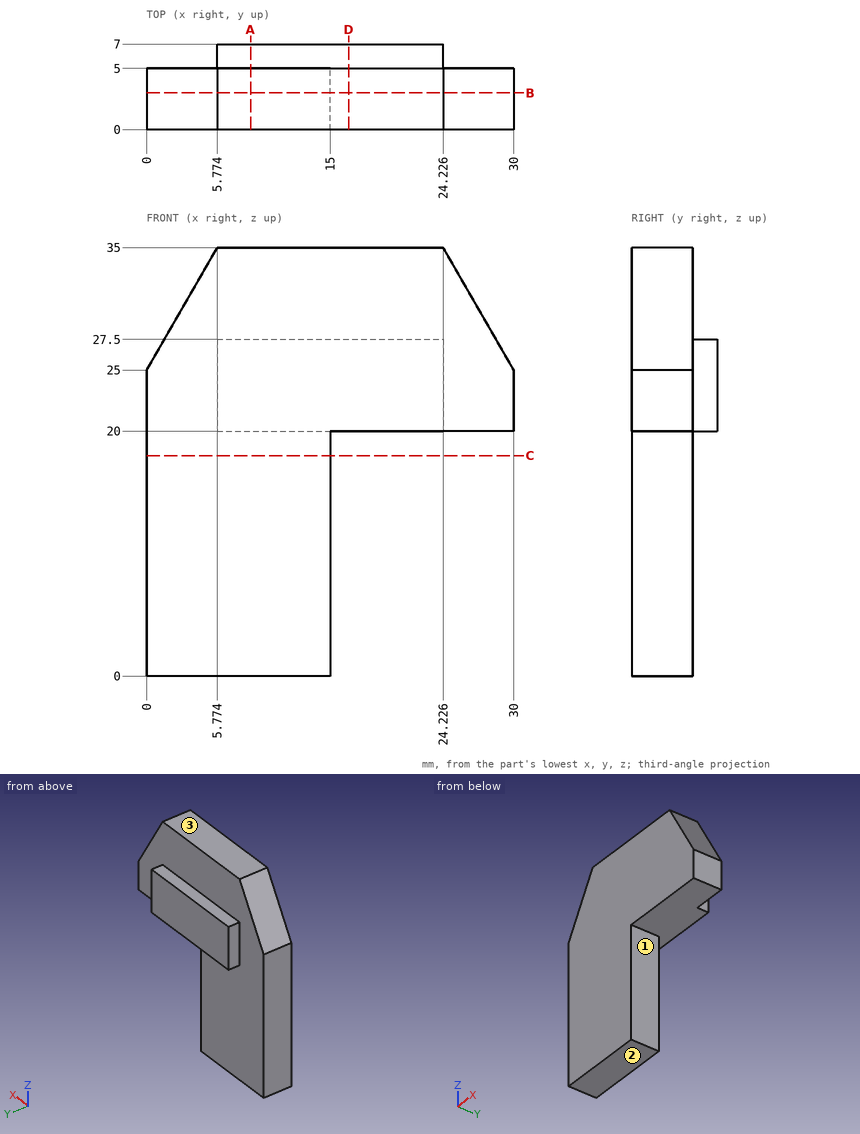
Verification items for this drawing (mm, ordinates from the low corner). Coordinates: 2 decimals unless noted, no trailing zeros. Order: outer loops, then holes, each group sorted by start corner. A loop starts at its lowest first (then second) coordinate and runs counter-clockwise, first axis right, second up. Notation, with made-up numbers: M 81,22 L 91,22 A18 ccw 91,57 Z; hole C 87.25,39.5 d7. An arc over 180 degrees is marked long. One line per item, written item: value. Start each with the question number.
Item 1: Thickness scan on probe 1 along Y at (x, z) = (2.25, 10); probe 2 along X at (y, z) = (2.75, 17); probe 3 along Z at (x, y) = (16.75, 6). Record the ranges inside material, lowest first.
Item 2: Sectioned sample at A-A on x = 8.5. Record the cut outline in (y, z), then the cut area to 3 significant figures.
Item 3: Sectioned sample at D-D on x = 16.5. Record the cut outline in (y, z).
Item 4: Sectioned sample at C-C on z = 18. Record the cut outline in (x, y), then the cut area to 3 significant figures.
Item 5: Depth check by flat-ended pin: P1, Ø9, axis at x = 16.5, z = 14.5, coming from the +Y side; P2, Ø0.6, axis at x = 18, y = 5.5, coming from the +Z side; P3, Ø2.5, axis at y = 2, z = 10.5, coming from the +X side. Enter the tip coordinate at first touch or a pass-through.
Item 6: Mould release check, pull along Z, two halves, no side actions. Record for the marked faces 1, 2 and 3: pulls with the +Z half, pulls with the -Z half, needs draft (parallel to the pull), parting line crosses it, or undercut.
Item 7: Sectioned sample at B-B on y = 3. Record the cut outline in (x, z).
Calculated:
1. probe 1: 0 to 5
1. probe 2: 0 to 15
1. probe 3: 20 to 27.5
2. outline: M 0,0 L 5,0 L 5,20 L 7,20 L 7,27.5 L 5,27.5 L 5,35 L 0,35 Z
2. area: 190 mm^2
3. outline: M 0,20 L 7,20 L 7,27.5 L 5,27.5 L 5,35 L 0,35 Z
4. outline: M 0,0 L 15,0 L 15,5 L 0,5 Z
4. area: 75.0 mm^2
5. P1: y = 5
5. P2: z = 27.5
5. P3: x = 15
6. face 1: needs draft
6. face 2: pulls with the -Z half
6. face 3: pulls with the +Z half
7. outline: M 0,0 L 15,0 L 15,20 L 30,20 L 30,25 L 24.23,35 L 5.77,35 L 0,25 Z
